Check sheet for the modelled part. Datum: model origin and axes. Units: mm. A direction names the side the tool comes from. Round coordinates to 2 decimals unless told otherwise and drop trailing zeros. Write each loop counter-clockwise with the first axis right and the second up, starting at its lowest first coordinate (ties: lowest second). Pieces come first, ordered by that corner, then holes. Notation, with made-up numbers: M 1.5,-21.75 L 41.5,-21.75 A29 ccw 41.5,8.25 Z; hole C -25,-14.5 d5. An arc over 180 degrees is marked long. Answer in a Markdown table with one row per item.
```python
from build123d import *

# Parameters (mm, degrees)
F0_W     = 1200
F0_H     = 1050
F1_DEPTH = 100
F2_W     = 150
F2_H     = 100
F3_DEPTH = 2300
F4_W     = 1200
F4_H     = 400
F5_DEPTH = 100


with BuildPart() as f1:
    # F0 (on Front) → F1 (new body)
    with BuildSketch(Plane.XZ):
        Rectangle(F0_W, F0_H)
    extrude(amount=F1_DEPTH)

    # F2 (on face) → F3 (join)
    with BuildSketch(Plane(origin=(0, 0, -525), x_dir=(1, 0, 0), z_dir=(0, 0, -1))):
        with Locations((675, 50)):
            Rectangle(F2_W, F2_H)
        with Locations((-675, 50)):
            Rectangle(F2_W, F2_H)
    extrude(amount=-F3_DEPTH)

    # F4 (on face) → F5 (join, through all)
    with BuildSketch(Plane.XZ.offset(100)):
        with Locations((0, 1575)):
            Rectangle(F4_W, F4_H)
    extrude(amount=-F5_DEPTH)


solid = f1.part
```
1. Section check A-A, the plane y = -83. Record the cut outline in (x, z), and give its area (3 significant figures).
Found:
| item | result |
|---|---|
| outline | M -750,-525 L 750,-525 L 750,1775 L -750,1775 Z; hole M -600,525 L 600,525 L 600,1375 L -600,1375 Z |
| area | 2,430,000 mm2 |
2. Draft check along Z on faces 1 (the face through (-8, -51, 1375)), 2 (the face through (-10, -51, -525)), 3 (the face through (750, -49, 609)), 4 (the face through (-8, -49, 525)). Enter one of: +Z half, -Z half, draft (parallel to the pull), parting line (faces both ways), or undercut.
Found:
| item | result |
|---|---|
| face 1 | undercut |
| face 2 | -Z half |
| face 3 | draft |
| face 4 | undercut |
3. Go/stop test with a flat-tipped pin: pin 1 (3 mm diameter, centred on x = -30, z = 111, fed in from +Y). Record where the tip stops, or that it passes through.
Found:
| item | result |
|---|---|
| pin 1 | stops at y = 0 |
4. Scan lines: L1, parallel to Z at x = 167, y = -73; L2, parallel to X at y = -61.5, z = 623.5. Record each from-to range of solid material in increasing order.
Found:
| item | result |
|---|---|
| L1 | z = -525 to 525, 1375 to 1775 |
| L2 | x = -750 to -600, 600 to 750 |
5. Section check B-B, the plane z = 652.5. Record the cut outline in (x, y), and give its area (3 significant figures).
Found:
| item | result |
|---|---|
| outline | M -750,-100 L -600,-100 L -600,0 L -750,0 Z; M 600,-100 L 750,-100 L 750,0 L 600,0 Z |
| area | 30,000 mm2 |
6. Access from +Z, -Z, +X, -X, +Y, -Y to the whole of each face (thin tool, end or side, straight path). Record for faces 5 (the face through (-600, -49, 944)), 6 (the face through (-10, -100, 386)).
Found:
| item | result |
|---|---|
| face 5 | +Y, -Y |
| face 6 | +Z, -Z, +X, -X, -Y |
7. Section check C-C, the plane x = -548. Record the cut outline in (y, z), and give its area (3 significant figures).
Found:
| item | result |
|---|---|
| outline | M -100,-525 L 0,-525 L 0,525 L -100,525 Z; M -100,1375 L 0,1375 L 0,1775 L -100,1775 Z |
| area | 145,000 mm2 |
